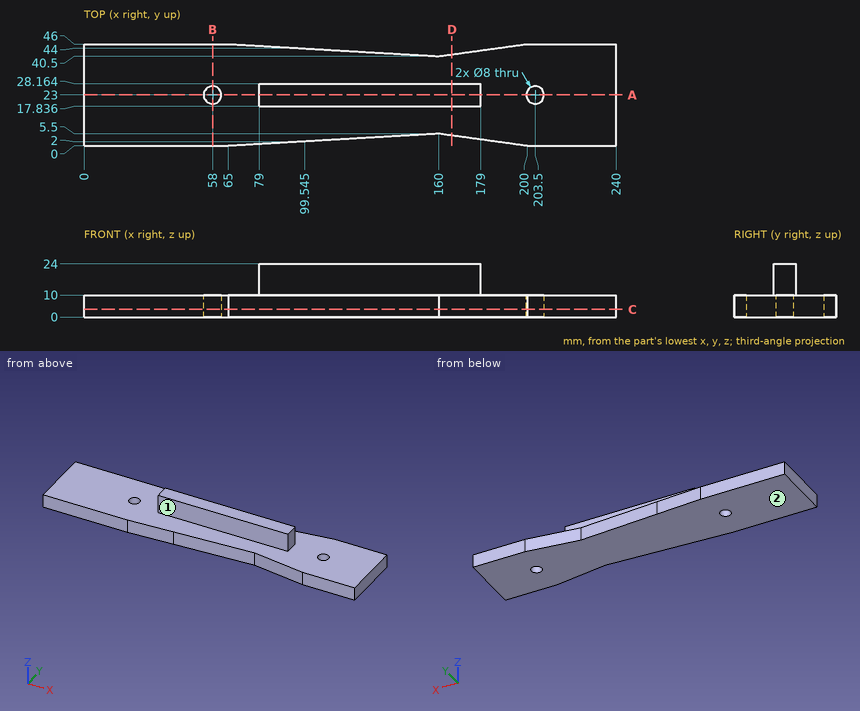
The drawing under review shows one solid part. Ordinate dimensions are in mm from its lowest x, y, z. A direction names the side the tool comes from. Round coordinates to 2 decimals unless told otherwise and drop trailing zeros. Loops run counter-clockwise (first coordinate to the right, second up) from the corner with the lowest first, then second, coordinate; pieces in that order, holes last. Notation, with made-up numbers: (12.25, -30) - (50.25, -30) arc R23 ccw to (50.25, -5) - close; hole circle Ø2 at (65, -2.5). An arc over 180 degrees is marked (long way). Put each result on its own line as item: value. Start each with the question number.
1. Insertion check: P1, Ø8.5, axis at y = 24.5, z = 20, coming from the +X side; P2, Ø8, axis at x = 45, y = 21.5, coming from the +Z side; P3, Ø6.5, axis at x = 203.5, y = 23, coming from the -Z side; P4, Ø5, axis at y = 21.5, z = 16, coming from the -X side. Each pin has a flat end and moves straight along its axis. Give the tip position at first contact, or say it passes through.
2. Consider section B-B on x = 58. State the section outline as (y, z) points.
3. Consider section D-D on x = 166. State the section outline as (y, z) points (1 decimal).
4. Consider section A-A on y = 23. State the section outline as (x, z) points.
5. Consider section C-C on z = 3.5. State the section outline as (x, y) points (1 decimal).
6. For probe 1 along Y at (x, z) = (203.5, 5.5); probe 2 along Y at (x, z) = (138.5, 13.75); probe 3 along Z at (x, y) = (38, 28), list the stretches that pass through material, from the lowest coordinate up. Write a range as [from, to].
7. For the marked faces 1 and 2, list the 3-axis set-ups (+Z, -Z, +X, -X, +Y, -Y) from which the entire face can be reached by the end or side of a thin tool; tool diameter is ignored.
Result sheet:
1. P1: x = 179
1. P2: z = 10
1. P3: through
1. P4: x = 79
2. outline: (0, 0) - (19, 0) - (19, 10) - (0, 10) - close; (27, 0) - (46, 0) - (46, 10) - (27, 10) - close
3. outline: (4.7, 0) - (41.3, 0) - (41.3, 10) - (28.2, 10) - (28.2, 24) - (17.8, 24) - (17.8, 10) - (4.7, 10) - close
4. outline: (0, 0) - (54, 0) - (54, 10) - (0, 10) - close; (62, 0) - (199.5, 0) - (199.5, 10) - (179, 10) - (179, 24) - (79, 24) - (79, 10) - (62, 10) - close; (207.5, 0) - (240, 0) - (240, 10) - (207.5, 10) - close
5. outline: (0, 0) - (65, 0) - (160, 5.5) - (200, 0) - (240, 0) - (240, 46) - (200, 46) - (160, 40.5) - (65, 46) - (0, 46) - close; hole circle Ø8 at (58, 23); hole circle Ø8 at (203.5, 23)
6. probe 1: [0, 19], [27, 46]
6. probe 2: [17.84, 28.16]
6. probe 3: [0, 10]
7. face 1: +Z, +X, -X, -Y
7. face 2: -Z, +X, -X, +Y, -Y
